Autodesk Inventor part; units mm, degrees
ref_plane "YZ Plane" through (0, 0, 0) normal (1, 0, 0) x (0, 1, 0)
ref_plane "XZ Plane" through (0, 0, 0) normal (0, 1, 0) x (-1, 0, 0)
ref_plane "XY Plane" through (0, 0, 0) normal (0, 0, 1) x (1, 0, 0)
sketch "Sketch1" plane through (0, 0, 0) normal (0, 0, 1) x (1, 0, 0)
  circle A0 centre (0, 0) radius 3.175
  arc A1 (0, -12.7) -> (0, 12.7) centre (0, 0) ccw
  line L0 (0, 12.7) -> (-9.525, 12.7)
  line L1 (0, -12.7) -> (-9.525, -12.7)
  line L2 (-9.525, 12.7) -> (-22.225, 12.7)
  line L3 (-22.225, -12.7) -> (-9.525, -12.7)
  line L4 (-22.225, 12.7) -> (0, 12.7)
  line L5 (0, -12.7) -> (-22.225, -12.7)
  circle A2 centre (-44.45, 0) radius 3.175
  arc A3 (-44.45, 12.7) -> (-44.45, -12.7) centre (-44.45, 0) ccw
  line L6 (-44.45, 12.7) -> (-34.925, 12.7)
  line L7 (-44.45, -12.7) -> (-34.925, -12.7)
  line L8 (-34.925, 12.7) -> (-22.225, 12.7)
  line L9 (-22.225, -12.7) -> (-34.925, -12.7)
  line L10 (-22.225, 12.7) -> (-44.45, 12.7)
  line L11 (-44.45, -12.7) -> (-22.225, -12.7)
  dimension "d0" = 6.35
  dimension "d5" = 25.4
  dimension "d6" = 12.7
extrude "Extrusion1" add sketch "Sketch1" along normal blind 3.175
properties part number "linear_slide_piece2_v2" material "Aluminum 6061"
For this review, take the finished solid that the model builds, in its own axes (mm). Round coordinates to 2 decimals unless told otherwise and drop trailing zeros. Write each loop counter-clockwise with the first axis right and the second up, starting at its lowest first coordinate (ties: lowest second). Pieces come first, ordered by that corner, then holes. Notation, with made-up numbers: (2, -11.5) -> (44, -11.5) arc R17 ccw to (44, -1.5) -> close; hole circle Ø1 at (86, 20.5). An arc over 180 degrees is marked (long way). Put each result on its own line as item: value.
Q1. Consider section C-C on y = 5.75. State the section outline as (x, z) points (3 decimals), and give its area (3 significant figures).
Determined:
outline: (-55.774, 0) -> (11.324, 0) -> (11.324, 3.175) -> (-55.774, 3.175) -> close
area: 213 mm^2
Q2. Consider section B-B on z = 0.55. State the section outline as (x, y) points (3 decimals).
Determined:
outline: (-44.45, -12.7) -> (0, -12.7) arc R12.7 ccw to (0, 12.7) -> (-44.45, 12.7) arc R12.7 ccw to start; hole circle Ø6.35 at (-44.45, 0); hole circle Ø6.35 at (0, 0)
Q3. The part is to be moulded in two halves that separate along Y. For faces 1 (the cylindrical face through (-0.69, 3.1, 1.57)), 2 (the flat face through (-23, -12.7, 2)), 3 (the flat face through (-23, 12.7, 2)), say which applies: released by +Y, released by -Y, zero draft, split by the parting line, or undercut.
Determined:
face 1: undercut
face 2: released by -Y
face 3: released by +Y
Q4. Consider section A-A on y = 0. State the section outline as (x, z) points (3 decimals), and give its area (3 significant figures).
Determined:
outline: (-57.15, 0) -> (-47.625, 0) -> (-47.625, 3.175) -> (-57.15, 3.175) -> close; (-41.275, 0) -> (-3.175, 0) -> (-3.175, 3.175) -> (-41.275, 3.175) -> close; (3.175, 0) -> (12.7, 0) -> (12.7, 3.175) -> (3.175, 3.175) -> close
area: 181 mm^2
Q5. Consider section D-D on y = -9. State the section outline as (x, z) points (3 decimals).
Determined:
outline: (-53.41, 0) -> (8.96, 0) -> (8.96, 3.175) -> (-53.41, 3.175) -> close
Q6. To check wall thickness, follow L1, parallel to X at y = 2.5, z = 1.5; L2, parallel to Y at x = -44.45, z = 1.4 (3 decimals); L3, parallel to Y at x = 0.5, z = 2.8. State the ranges of each line that lie inside material, in increasing order. Write a range as [from, to].
Determined:
L1: x = [-56.9, -46.41], [-42.49, -1.96], [1.96, 12.45]
L2: y = [-12.7, -3.175], [3.175, 12.7]
L3: y = [-12.69, -3.14], [3.14, 12.69]
